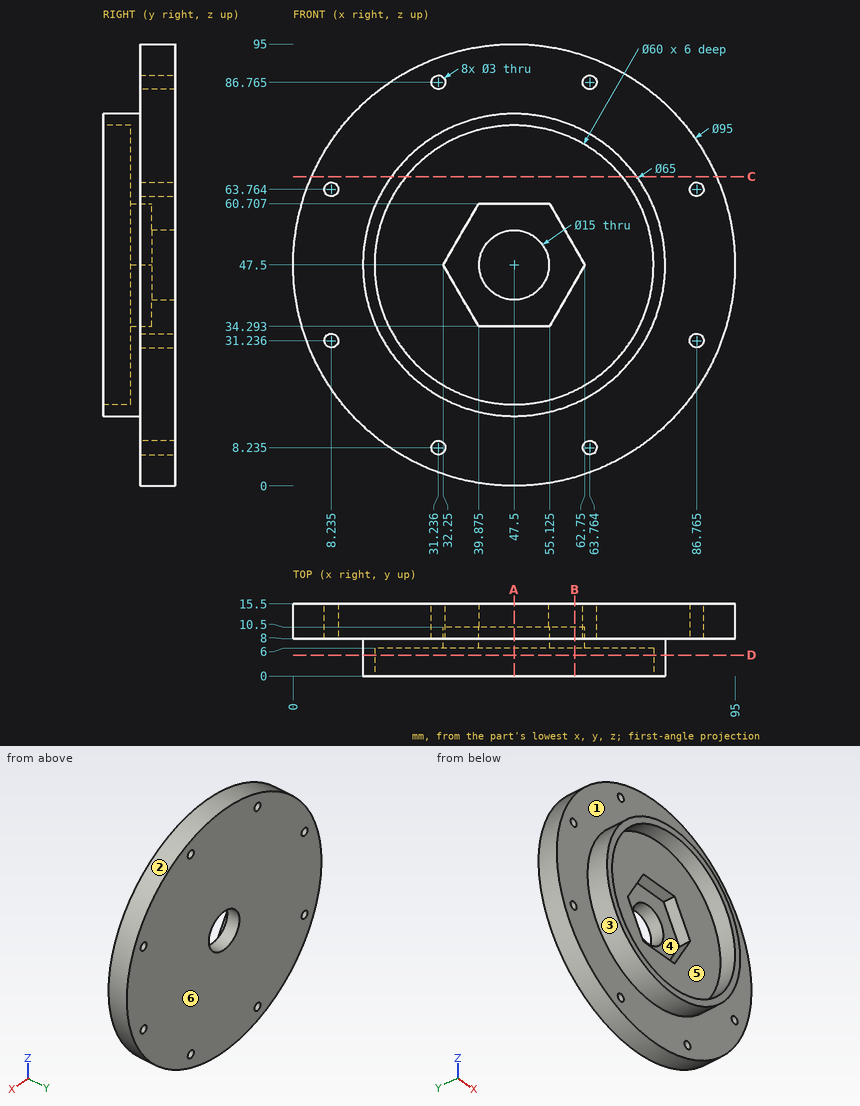
Part print with two shaded views. Sizes in mm from the minimum x, y, z corner. A direction names the side the tool comes from. Give positions to 0.01 mm unless a question says otherwise; leave off trailing zeros. Order: outer loops, then holes, each group sorted by start corner. A loop starts at its lowest first (then second) coordinate and runs counter-clockwise, first axis right, second up. Notation, with made-up numbers: M 65.5,68.25 L 122.5,68.25 A19 cw 122.5,85.25 Z; hole C 13,46.25 d2. An arc over 180 degrees is marked long. Write item = value, one per line.
Q1. Cut at A-A, the plane x = 47.5. List the corners of the cut face in (y, z).
Derived:
outline = M 0,15 L 8,15 L 8,0 L 15.5,0 L 15.5,40 L 10.5,40 L 10.5,34.29 L 6,34.29 L 6,17.5 L 0,17.5 Z; M 0,77.5 L 6,77.5 L 6,60.71 L 10.5,60.71 L 10.5,55 L 15.5,55 L 15.5,95 L 8,95 L 8,80 L 0,80 Z
Q2. Flat gauge pins, fed straight in: pin 1 (2.5 mm diameter, centred on x = 86.76, z = 31.24, fed in from -Y); pin 2 (5 mm diameter, centred on x = 76.5, z = 14, fed in from -Y); pin 3 (19.5 mm diameter, centred on x = 47.5, z = 47.5, fed in from -Y); pin 4 (3.5 mm diameter, centred on x = 49.5, y = 7.5, fed in from -Z). Where does each tip first touch, or does it go through?
Derived:
pin_1 = through
pin_2 = 8
pin_3 = 10.5
pin_4 = 0
Q3. Cut at C-C, the plane z = 66.5. List the corners of the cut face in (x, y), then the cut area to 3 significant figures.
Derived:
outline = M 3.97,8 L 21.13,8 L 21.13,0 L 24.28,0 L 24.28,6 L 70.72,6 L 70.72,0 L 73.87,0 L 73.87,8 L 91.03,8 L 91.03,15.5 L 3.97,15.5 Z
area = 796 mm2
Q4. Two-plate mould, pull along X, no slides. Class the marked faces 3, 4, 5 and 6: pulls with the +X half, pulls with the -X half, needs draft (parallel to the pull), parting line crosses it, or undercut.
Derived:
face_3 = parting line crosses it
face_4 = undercut
face_5 = undercut
face_6 = needs draft
Q5. Drill centre lines: line 1 (X direction, y = 14, z = 47.5); line 2 (Y direction, x = 38.5, z = 61); line 3 (Y direction, x = 60.5, z = 7). Where is each one in solid material? Low to high. Write a range as [from, to].
Derived:
line_1 = [0, 40], [55, 95]
line_2 = [6, 15.5]
line_3 = [8, 15.5]
Q6. Tool access for the marked faces 1 and 2: list every direction of +Z, -Z, +X, -X, +Y, -Y with a clear straight run to the whole face (end or side of a thin tool).
Derived:
face_1 = -Y
face_2 = +Y, -Y
Q7. Cut at B-B, the plane x = 60.5. List the corners of the cut face in (y, z), then the cut area to 3 significant figures.
Derived:
outline = M 0,17.71 L 8,17.71 L 8,1.81 L 15.5,1.81 L 15.5,93.19 L 8,93.19 L 8,77.29 L 0,77.29 L 0,74.54 L 6,74.54 L 6,51.4 L 10.5,51.4 L 10.5,43.6 L 6,43.6 L 6,20.46 L 0,20.46 Z
area = 802 mm2
Q8. Cut at D-D, the plane y = 4.5. List the corners of the cut face in (x, z).
Derived:
outline = C 47.5,47.5 d65; hole C 47.5,47.5 d60
